from build123d import *

# Parameters (mm, degrees)
PAD_DEPTH    = 140
SKETCH001_R  = 2.5
POCKET_DEPTH = 16.001


with BuildPart() as part:
    # Sketch → Pad (new body, symmetric)
    with BuildSketch(Plane.XZ):
        Polygon((0, 0), (0, 16), (16, 16), (16, 0), (14, 0), (14, 14), (2, 14), (2, 0), align=None)
    extrude(amount=PAD_DEPTH, both=True)

    # Sketch001 → Pocket (cut, through all)
    with BuildSketch(Plane(origin=(16, 0, 0), x_dir=(0, 0, 1), z_dir=(1, 0, 0))):
        with Locations((7, 130)):
            Circle(SKETCH001_R)
        with Locations((7, -130)):
            Circle(SKETCH001_R)
        with Locations((7, 24)):
            Circle(SKETCH001_R)
        with Locations((7, -30)):
            Circle(SKETCH001_R)
    extrude(amount=-POCKET_DEPTH, mode=Mode.SUBTRACT)


solid = part.part
Here's how the part is built. I have some questions about the finished solid (model axes, mm). A direction names the side the tool comes from. Coordinates: 2 decimals unless noted, no trailing zeros. Order: outer loops, then holes, each group sorted by start corner. A loop starts at its lowest first (then second) coordinate and runs counter-clockwise, first axis right, second up.
Item 1: If we mould it in two halves opening along X, with no side actions, what happens to faces 3 (the face through (8, -2, 14)), 4 (the face through (0, -2, 8)), 5 (the face through (14, -2, 7)), 6 (the face through (16, -2, 8))? For each: +X half, -X half, draft (parallel to the pull), parting line (faces both ways), or undercut.
Result sheet:
face 3: undercut
face 4: -X half
face 5: undercut
face 6: +X half
Item 2: If we section it at B-B on y = -52: List the corners of the cut face in (x, z) for me, plus the area to 3 significant figures.
Result sheet:
outline: (0, 0) - (2, 0) - (2, 14) - (14, 14) - (14, 0) - (16, 0) - (16, 16) - (0, 16) - close
area: 88.0 mm2
Item 3: For faces 1 (the face through (1.01, 127.52, 6.67)), 2 (the face through (2, -2, 7)), which set-ups out of +Z, -Z, +X, -X, +Y, -Y let a thin tool reach every point of the face, with its end or its side?
Result sheet:
face 1: +X, -X
face 2: -Z, +Y, -Y
Item 4: For P1, Ø4, axis at y = 130, z = 7, coming from the +X side; P2, Ø2, axis at x = 7.5, y = 102, coming from the -Z side, each with a flat end and sliding along its axis, tell me the tip position at first contact or that it passes through.
Result sheet:
P1: passes through
P2: stops at z = 14
Item 5: If we section it at C-C on z = 7: State how many separate pieces and enclosed holes the cut face has, plus the area to 3 significant figures.
Result sheet:
separate pieces: 10
enclosed holes: 0
area: 1,040 mm2
Item 6: If we section it at D-D on x = 5.5: List the corners of the cut face in (y, z) for me.
Result sheet:
outline: (-140, 14) - (140, 14) - (140, 16) - (-140, 16) - close
Item 7: If we section it at A-A on y = -130: List the corners of the cut face in (x, z) for me, plus the area to 3 significant figures.
Result sheet:
outline: (0, 0) - (2, 0) - (2, 4.5) - (0, 4.5) - close; (0, 9.5) - (2, 9.5) - (2, 14) - (14, 14) - (14, 9.5) - (16, 9.5) - (16, 16) - (0, 16) - close; (14, 0) - (16, 0) - (16, 4.5) - (14, 4.5) - close
area: 68.0 mm2
Item 8: I need wall thicknesses on line 1 (Y direction, x = 15.3, z = 7); line 2 (X direction, y = 69.5, z = 10.75); line 3 (Z direction, x = 14.55, y = -24). Which ranges of each line are inside material? Lowest first, please.
Result sheet:
line 1: y = -140 to -132.5, -127.5 to -26.5, -21.5 to 27.5, 32.5 to 127.5, 132.5 to 140
line 2: x = 0 to 2, 14 to 16
line 3: z = 0 to 4.5, 9.5 to 16
